Can you work these out from the drawing? Everything is in mm from the part's minimum corner. A direction names the side the tool comes from. Coordinates: 2 decimals unless noted, no trailing zeros. Answer as a JSON object with one key per item and string values.
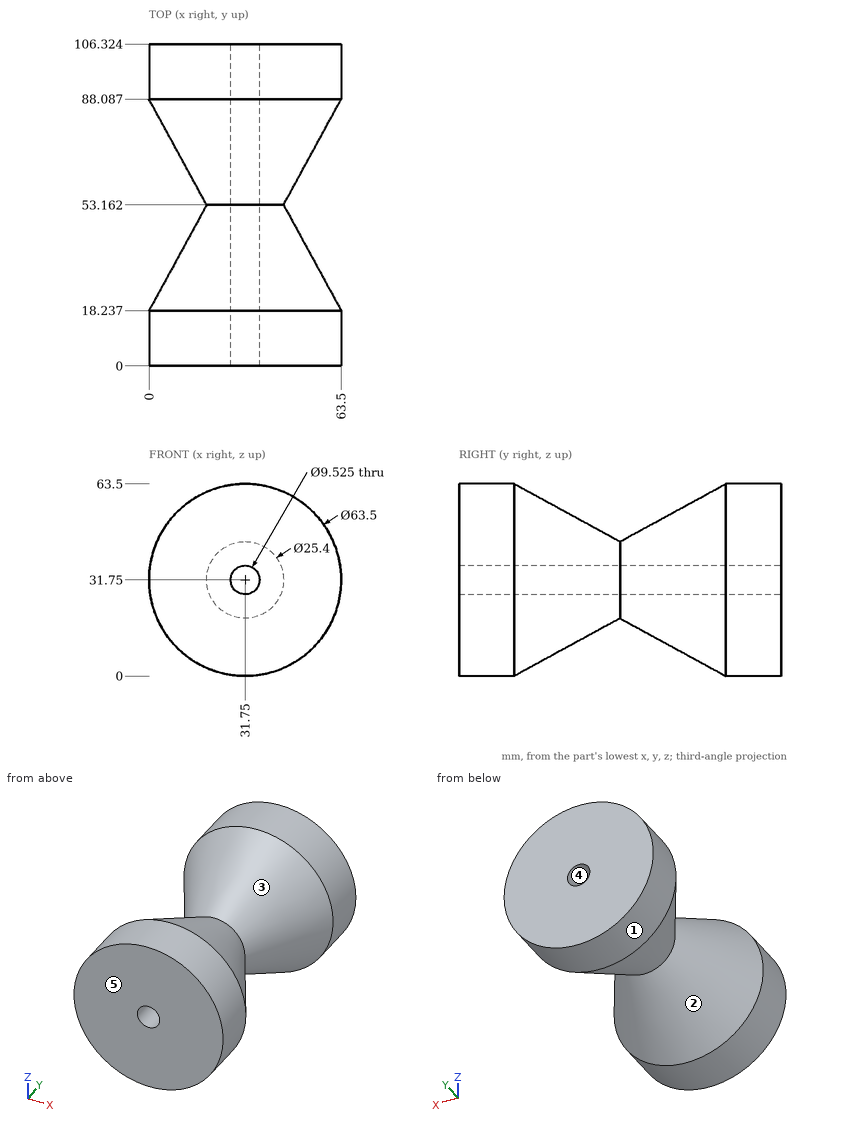
Item 1: If we mould it in two halves opening along Z, with no side actions, what happens to the marked faces 3, 4 and 5? For each: pulls with the +Z half, pulls with the -Z half, needs draft (parallel to the pull), parting line crosses it, or undercut.
Answers follow:
{"face 3": "parting line crosses it", "face 4": "undercut", "face 5": "needs draft"}
Item 2: Which directions (+Z, -Z, +X, -X, +Y, -Y) give clear straight access to the entire face, cutting with the end or side of a thin tool? Please do the marked faces 1 and 2.
Answers follow:
{"face 1": "+Y, -Y", "face 2": "none"}
Item 3: Please list where these lines run through material, in increasing order: line 1 (Z direction, x = 31.75, y = 25); line 2 (X direction, y = 19.5, z = 31); line 3 (Z direction, x = 31.75, y = 68.5) (1 decimal).
Answers follow:
{"line 1": "z = 3.69 to 26.99, 36.51 to 59.81", "line 2": "x = 0.7 to 27.05, 36.45 to 62.8", "line 3": "z = 10.7 to 27, 36.5 to 52.8"}
Item 4: I'm going to push flat-ended pins straight in: pin 1 (5 mm diameter, centred on y = 88.5, z = 36.5, fed in from +X); pin 2 (6 mm diameter, centred on y = 25, z = 46.5, fed in from +X); pin 3 (10 mm diameter, centred on x = 46, y = 17.5, fed in from +Z); pin 4 (5.5 mm diameter, centred on x = 31.75, z = 31.75, fed in from -Y). Where does each tip first touch, or does it pass through?
Answers follow:
{"pin 1": "stops at x = 63.42", "pin 2": "stops at x = 58.11", "pin 3": "stops at z = 62.12", "pin 4": "passes through"}
